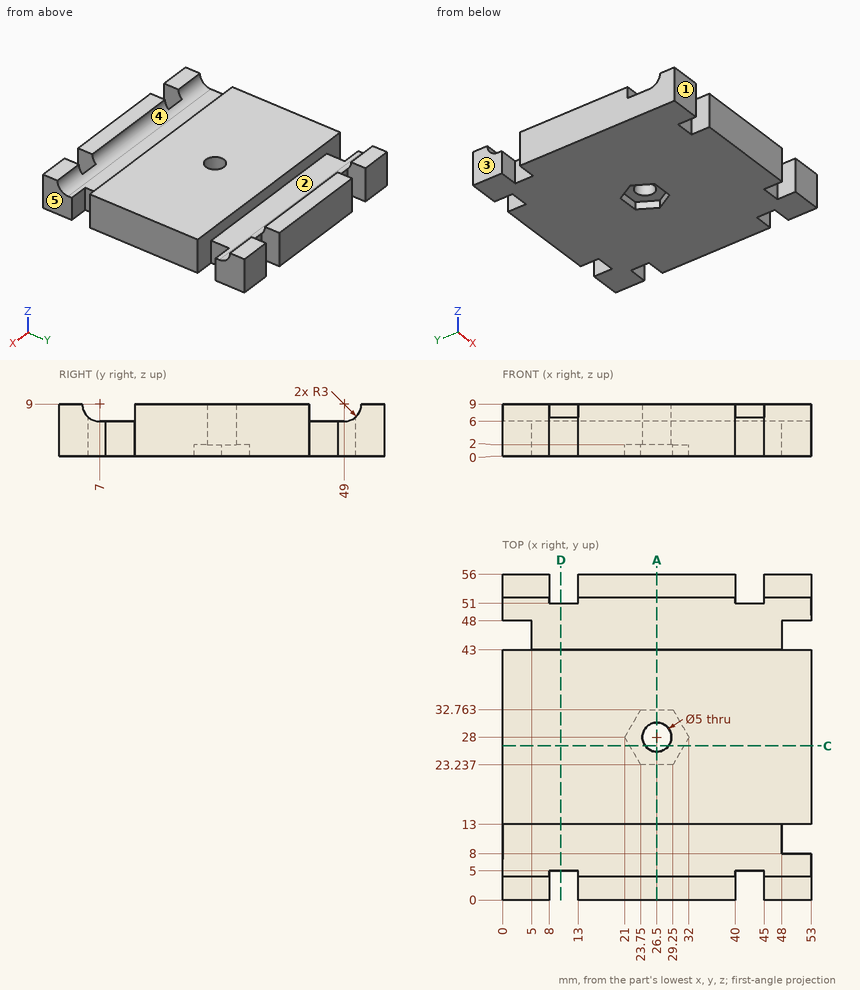
Study the drawing (mm; zero at the part's minimum x, y, z) and answer. A direction names the side the tool comes from. Give positions to 0.01 mm unless a question says otherwise; leave off trailing zeros. Write each loop counter-clockwise with the first axis right and the second up, starting at its lowest first coordinate (ties: lowest second). Pieces come first, ordered by that corner, then holes.
(1) Straight lines are drawn through the part: line 1 (X direction, y = 28, z = 4); line 2 (X direction, y = 4.5, z = 4.25); line 3 (Y direction, x = 26.5, z = 4.5). For each, find the intervals that lie inside material, in ascending order.
Final values:
line 1: x = 0 to 24, 29 to 53
line 2: x = 0 to 8, 13 to 40, 45 to 53
line 3: y = 0 to 25.5, 30.5 to 56
(2) Which of the six approach directions +Z, -Z, +X, -X, +Y, -Y give full straight-line access (tool end or side, diameter ignored) to the marked faces 4 and 5?
Final values:
face 4: +Z, +X, -X
face 5: +Z, -Z, +X, +Y, -Y
(3) Flat-ended cylindrical pins translate along their axes: pin 1 Ø6.5 at (x, y) = (30.5, 9) entering from +Z; pin 2 Ø8 at (x, y) = (26.5, 28) entering from -Z; pin 3 Ø2.5 at (x, z) = (42, 2.5) entering from -Y. Find the tip coordinate at first contact, or state that the pin passes through.
Final values:
pin 1: stops at z = 6.27
pin 2: stops at z = 2
pin 3: stops at y = 5
(4) The part is cut by section C-C on y = 26.5. Write down the section's boundary in (x, z).
Final values:
outline: (0, 0) - (21.87, 0) - (21.87, 2) - (24.5, 2) - (24.5, 9) - (0, 9) - close; (28.5, 2) - (31.13, 2) - (31.13, 0) - (53, 0) - (53, 9) - (28.5, 9) - close
(5) The mould has two halves that part along Y. Classify the marked faces 1, 2 and 3: pulls with the +Y half, pulls with the -Y half, needs draft (parallel to the pull), parting line crosses it, or undercut.
Final values:
face 1: pulls with the -Y half
face 2: undercut
face 3: needs draft
(6) The part is cut by section A-A on x = 26.5. Write down the section's boundary in (y, z), plus the area to 3 significant figures.
Final values:
outline: (0, 0) - (23.24, 0) - (23.24, 2) - (25.5, 2) - (25.5, 9) - (13, 9) - (13, 6) - (7, 6) arc R3 cw to (4, 9) - (0, 9) - close; (30.5, 2) - (32.76, 2) - (32.76, 0) - (56, 0) - (56, 9) - (52, 9) arc R3 cw to (49, 6) - (43, 6) - (43, 9) - (30.5, 9) - close
area: 400 mm2
(7) The part is cut by section D-D on x = 10. Write down the section's boundary in (y, z).
Final values:
outline: (5, 0) - (51, 0) - (51, 6.76) arc R3 cw to (49, 6) - (43, 6) - (43, 9) - (13, 9) - (13, 6) - (7, 6) arc R3 cw to (5, 6.76) - close
